For this review, take the finished solid that the model builds, in its own axes (mm). Give positions to 0.01 mm unless a question says otherwise; leave off trailing zeros. Answer as CSV lines item,"result".
```python
from build123d import *

# Parameters (mm, degrees)
BR_EXTRUDE_DEPTH      = 160
BR_EXTRUDE_DEPTH_BACK = 160


with BuildPart() as part:
    # Sketch2 → BR_Extrude (new body, two sides)
    with BuildSketch(Plane(origin=(0, 0, 0), x_dir=(0, 0, -1), z_dir=(1, 0, 0))) as br_extrude_sk:
        with BuildLine():
            Line((-6, 4.196877708), (-10.053122292, 8.25))
            Line((-10.053122292, 8.25), (-12.8, 8.25))
            Line((-12.8, 8.25), (-12.800036742, 4.05))
            Line((-12.800036742, 4.05), (-14.5, 4.05))
            Line((-14.5, 4.05), (-14.5, 4.55))
            Line((-14.5, 4.55), (-15, 4.55))
            Line((-15, 4.55), (-15, 13))
            ThreePointArc((-15, 13), (-14.414213562, 14.414213562), (-13, 15))
            Line((-13, 15), (-4.55, 15))
            Line((-4.55, 15), (-4.55, 14.5))
            Line((-4.55, 14.5), (-4.05, 14.5))
            Line((-4.05, 14.5), (-4.05, 12.800036742))
            Line((-4.05, 12.800036742), (-8.25, 12.8))
            Line((-8.25, 12.8), (-8.25, 10.053122292))
            Line((-8.25, 10.053122292), (-4.196877708, 6))
            Line((-4.196877708, 6), (4.196877708, 6))
            Line((4.196877708, 6), (8.25, 10.053122292))
            Line((8.25, 10.053122292), (8.25, 12.8))
            Line((8.25, 12.8), (4.05, 12.800036742))
            Line((4.05, 12.800036742), (4.05, 14.5))
            Line((4.05, 14.5), (4.55, 14.5))
            Line((4.55, 14.5), (4.55, 15))
            Line((4.55, 15), (13, 15))
            ThreePointArc((13, 15), (14.414213562, 14.414213562), (15, 13))
            Line((15, 13), (15, 4.55))
            Line((15, 4.55), (14.5, 4.55))
            Line((14.5, 4.55), (14.5, 4.05))
            Line((14.5, 4.05), (12.800036742, 4.05))
            Line((12.800036742, 4.05), (12.8, 8.25))
            Line((12.8, 8.25), (10.053122292, 8.25))
            Line((10.053122292, 8.25), (6, 4.196877708))
            Line((6, 4.196877708), (6, -4.196877708))
            Line((6, -4.196877708), (10.053122292, -8.25))
            Line((10.053122292, -8.25), (12.8, -8.25))
            Line((12.8, -8.25), (12.800036742, -4.05))
            Line((12.800036742, -4.05), (14.5, -4.05))
            Line((14.5, -4.05), (14.5, -4.55))
            Line((14.5, -4.55), (15, -4.55))
            Line((15, -4.55), (15, -13))
            ThreePointArc((15, -13), (14.414213562, -14.414213562), (13, -15))
            Line((13, -15), (4.55, -15))
            Line((4.55, -15), (4.55, -14.5))
            Line((4.55, -14.5), (4.05, -14.5))
            Line((4.05, -14.5), (4.05, -12.800036742))
            Line((4.05, -12.800036742), (8.25, -12.8))
            Line((8.25, -12.8), (8.25, -10.053122292))
            Line((8.25, -10.053122292), (4.196877708, -6))
            Line((4.196877708, -6), (-4.196877708, -6))
            Line((-4.196877708, -6), (-8.25, -10.053122292))
            Line((-8.25, -10.053122292), (-8.25, -12.8))
            Line((-8.25, -12.8), (-4.05, -12.800036742))
            Line((-4.05, -12.800036742), (-4.05, -14.5))
            Line((-4.05, -14.5), (-4.55, -14.5))
            Line((-4.55, -14.5), (-4.55, -15))
            Line((-4.55, -15), (-13, -15))
            ThreePointArc((-13, -15), (-14.414213562, -14.414213562), (-15, -13))
            Line((-15, -13), (-15, -4.55))
            Line((-15, -4.55), (-14.5, -4.55))
            Line((-14.5, -4.55), (-14.5, -4.05))
            Line((-14.5, -4.05), (-12.800036742, -4.05))
            Line((-12.800036742, -4.05), (-12.8, -8.25))
            Line((-12.8, -8.25), (-10.053122292, -8.25))
            Line((-10.053122292, -8.25), (-6, -4.196877708))
            Line((-6, -4.196877708), (-6, 4.196877708))
        make_face()
        with BuildLine():
            Line((-13.85, -9.7), (-13.85, -12.85))
            ThreePointArc((-13.85, -12.85), (-13.557106781, -13.557106781), (-12.85, -13.85))
            Line((-12.85, -13.85), (-9.7, -13.85))
            Line((-9.7, -13.85), (-9.7, -9.7))
            Line((-9.7, -9.7), (-13.85, -9.7))
        make_face(mode=Mode.SUBTRACT)
        with BuildLine():
            Line((9.7, -13.85), (12.85, -13.85))
            ThreePointArc((12.85, -13.85), (13.557106781, -13.557106781), (13.85, -12.85))
            Line((13.85, -12.85), (13.85, -9.7))
            Line((13.85, -9.7), (9.7, -9.7))
            Line((9.7, -9.7), (9.7, -13.85))
        make_face(mode=Mode.SUBTRACT)
        with BuildLine():
            Line((13.85, 9.7), (13.85, 12.85))
            ThreePointArc((13.85, 12.85), (13.557106781, 13.557106781), (12.85, 13.85))
            Line((12.85, 13.85), (9.7, 13.85))
            Line((9.7, 13.85), (9.7, 9.7))
            Line((9.7, 9.7), (13.85, 9.7))
        make_face(mode=Mode.SUBTRACT)
        with BuildLine():
            Line((-9.7, 13.85), (-12.85, 13.85))
            ThreePointArc((-12.85, 13.85), (-13.557106781, 13.557106781), (-13.85, 12.85))
            Line((-13.85, 12.85), (-13.85, 9.7))
            Line((-13.85, 9.7), (-9.7, 9.7))
            Line((-9.7, 9.7), (-9.7, 13.85))
        make_face(mode=Mode.SUBTRACT)
        with BuildLine():
            Line((-3.272394192, -1.616767223), (-4.59052283, -3.187651763))
            Line((-4.59052283, -3.187651763), (-3.187651763, -4.59052283))
            Line((-3.187651763, -4.59052283), (-1.616767223, -3.272394192))
            ThreePointArc((-1.616767223, -3.272394192), (0, -3.65), (1.616767223, -3.272394192))
            Line((1.616767223, -3.272394192), (3.187651763, -4.59052283))
            Line((3.187651763, -4.59052283), (4.59052283, -3.187651763))
            Line((4.59052283, -3.187651763), (3.272394192, -1.616767223))
            ThreePointArc((3.272394192, -1.616767223), (3.65, 0), (3.272394192, 1.616767223))
            Line((3.272394192, 1.616767223), (4.59052283, 3.187651763))
            Line((4.59052283, 3.187651763), (3.187651763, 4.59052283))
            Line((3.187651763, 4.59052283), (1.616767223, 3.272394192))
            ThreePointArc((1.616767223, 3.272394192), (0, 3.65), (-1.616767223, 3.272394192))
            Line((-1.616767223, 3.272394192), (-3.187651763, 4.59052283))
            Line((-3.187651763, 4.59052283), (-4.59052283, 3.187651763))
            Line((-4.59052283, 3.187651763), (-3.272394192, 1.616767223))
            ThreePointArc((-3.272394192, 1.616767223), (-3.65, 0), (-3.272394192, -1.616767223))
        make_face(mode=Mode.SUBTRACT)
    extrude(amount=BR_EXTRUDE_DEPTH)
    extrude(br_extrude_sk.sketch, amount=-BR_EXTRUDE_DEPTH_BACK)


solid = part.part
```
Q1. Add section A-A (x = 22.5). State how many separate pieces and enclosed holes the cut face has, plus the area to 3 significant figures.
Answer block:
separate pieces,"1"
enclosed holes,"5"
area,"314 mm2"
Q2. Clearance check with flat-ended pins moving along their axes: pin 1 (1.4 mm diameter, centred on x = -16, z = -14, fed in from -Y); pin 2 (5 mm diameter, centred on x = 98, y = 0, fed in from +Z); pin 3 (0.6 mm diameter, centred on x = 55, z = -15, fed in from -Y). State where each tip first meets the part, or that it passes through.
Answer block:
pin 1,"stops at y = -14.98"
pin 2,"stops at z = 6"
pin 3,"stops at y = -14.05"
Q3. To check wall thickness, follow probe 1 along Z at (x, y) = (144.5, 12.25); probe 2 along Z at (x, y) = (98.5, -8). State the ranges of each line that lie inside material, in increasing order. Write a range as [from, to].
Answer block:
probe 1,"z = [-15, -13.85], [-9.7, -8.25], [8.25, 9.7], [13.85, 15]"
probe 2,"z = [-15, -12.8], [-9.8, -6.2], [6.2, 9.8], [12.8, 15]"
